from build123d import *

# Parameters (mm, degrees)
SKETCH1_W           = 38.1
SKETCH1_H           = 127
SKETCH1_R           = 4
SKETCH1_R_2         = 2.5
BOSS_EXTRUDE1_DEPTH = 4.7625


with BuildPart() as part:
    # Sketch1 → Boss-Extrude1 (new body)
    with BuildSketch(Plane.XY):
        with Locations((19.05, 63.5)):
            Rectangle(SKETCH1_W, SKETCH1_H)
        with Locations(Location((19.05, 25.4, 0), (0, 0, 180))):
            Circle(SKETCH1_R, mode=Mode.SUBTRACT)
        with Locations(Location((19.05, 6.9, 0), (0, 0, 180))):
            Circle(SKETCH1_R_2, mode=Mode.SUBTRACT)
        with Locations(Location((19.05, 43.9, 0), (0, 0, 180))):
            Circle(SKETCH1_R_2, mode=Mode.SUBTRACT)
    extrude(amount=BOSS_EXTRUDE1_DEPTH)


solid = part.part
Work out the finished part from the listing and answer in its coordinate system (mm). Coordinates: 2 decimals unless noted, no trailing zeros. Write each loop counter-clockwise with the first axis right and the second up, starting at its lowest first coordinate (ties: lowest second). Pieces come first, ordered by that corner, then holes. Notation, with made-up numbers: M -36.75,12 L -29.75,12 A16 ccw -29.75,27 Z; hole C 49.5,21.25 d4. An arc over 180 degrees is marked long. Use one line per item in the form item = value. Start each with the question number.
1. This flat-tipped pin is pushed along its axis until it touches: P1, Ø6.5, axis at x = 19.05, y = 25.4, coming from the -Z side. Where does it stop, or does it pass through?
2. Straight lines are drawn through the part: probe 1 along Y at (x, z) = (19.05, 3.6); probe 2 along X at (y, z) = (43.9, 3.85); probe 3 along X at (y, z) = (28.5, 1.7). For each, find the intervals that lie inside material, in ascending order. Write a range as from..to.
3. The mould has two halves that part along X. Classify faces 1 (the face through (19, 64, 4.762)), 2 (the face through (0, 63, 2)), 3 (the face through (17.71, 4.79, 2.35)): released by +X, released by -X, zero draft, split by the parting line, or undercut.
4. The part is cut by section A-A (y = 43.9). Give the vertices of the cut face in (x, z).
5. The part is cut by section D-D (y = 25.4). Give the vertices of the cut face in (x, z), plus the area to 3 significant figures.
6. The part is cut by section B-B (x = 19.05). Give the vertices of the cut face in (y, z).
7. The part is cut by section C-C (z = 0.75). Give the vertices of the cut face in (x, y), plus the area to 3 significant figures.
Evaluation:
q1.P1 = through
q2.probe_1 = 0..4.4, 9.4..21.4, 29.4..41.4, 46.4..127
q2.probe_2 = 0..16.55, 21.55..38.1
q2.probe_3 = 0..16.52, 21.58..38.1
q3.face_1 = zero draft
q3.face_2 = released by -X
q3.face_3 = undercut
q4.outline = M 0,0 L 16.55,0 L 16.55,4.76 L 0,4.76 Z; M 21.55,0 L 38.1,0 L 38.1,4.76 L 21.55,4.76 Z
q5.outline = M 0,0 L 15.05,0 L 15.05,4.76 L 0,4.76 Z; M 23.05,0 L 38.1,0 L 38.1,4.76 L 23.05,4.76 Z
q5.area = 143 mm^2
q6.outline = M 0,0 L 4.4,0 L 4.4,4.76 L 0,4.76 Z; M 9.4,0 L 21.4,0 L 21.4,4.76 L 9.4,4.76 Z; M 29.4,0 L 41.4,0 L 41.4,4.76 L 29.4,4.76 Z; M 46.4,0 L 127,0 L 127,4.76 L 46.4,4.76 Z
q7.outline = M 0,0 L 38.1,0 L 38.1,127 L 0,127 Z; hole C 19.05,25.4 d8; hole C 19.05,6.9 d5; hole C 19.05,43.9 d5
q7.area = 4,750 mm^2
